from build123d import *

# Parameters (mm, degrees)
F1_DEPTH = 38.1
F3_DEPTH = 28.448
F4_R     = 7.112
F5_DEPTH = 27.178
F6_R     = 8.001
F7_DEPTH = 28.448


with BuildPart() as f1:
    # F0 (on Top) → F1 (new body)
    with BuildSketch(Plane.XY):
        Polygon((-15.113, 0), (0, 0), (15.113, 0), (15.113, -38.1), (20.574, -38.1), (20.574, -53.848), (28.448, -53.848), (28.448, 11.43), (12.7, 27.178), (0, 27.178), (-12.7, 27.178), (-28.448, 11.43), (-28.448, -53.848), (-20.574, -53.848), (-20.574, -38.1), (-15.113, -38.1), align=None)
    extrude(amount=F1_DEPTH)

    # F2 (on Right) → F3 (cut, symmetric)
    with BuildSketch(Plane.YZ):
        Polygon((27.178, 38.1), (11.43, 38.1), (27.178, 29.0068), align=None)
        Polygon((27.178, 9.0932), (11.43, 0), (27.178, 0), align=None)
    extrude(amount=F3_DEPTH, both=True, mode=Mode.SUBTRACT)

    # F4 (on face) → F5 (cut)
    with BuildSketch(Plane(origin=(0, 27.178, 0), x_dir=(-1, 0, 0), z_dir=(0, 1, 0))):
        with Locations((0, 19.05)):
            Circle(F4_R)
    extrude(amount=-F5_DEPTH, mode=Mode.SUBTRACT)

    # F6 (on Right) → F7 (cut, symmetric)
    with BuildSketch(Plane.YZ):
        with Locations((-22.352, 19.05)):
            Circle(F6_R)
        with BuildLine():
            ThreePointArc((-53.848, 23.876), (-39.346733, 33.748623), (-22.352, 38.1))
            Line((-22.352, 38.1), (-53.848, 38.1))
            Line((-53.848, 38.1), (-53.848, 23.876))
        make_face()
    extrude(amount=F7_DEPTH, both=True, mode=Mode.SUBTRACT)


solid = f1.part
Build history of the part. All positions in model axes, mm. A direction names the side the tool comes from. Coordinates: 2 decimals unless noted, no trailing zeros. Order: outer loops, then holes, each group sorted by start corner. A loop starts at its lowest first (then second) coordinate and runs counter-clockwise, first axis right, second up. Notation, with made-up numbers: (-40, -11) -> (-33, -11) arc R14 ccw to (-33, -2) -> close; hole circle Ø3 at (78.25, 88). An arc over 180 degrees is marked (long way). One line per item, written item: value.
(1) Tool access for faces 4 (the flat face through (20.574, -46, 17)), 5 (the flat face through (-25, -53.848, 12)): list every direction of +Z, -Z, +X, -X, +Y, -Y with a clear straight run to the whole face (end or side of a thin tool).
Checked values:
face 4: +Z, -Z, -Y
face 5: +Z, -Z, +X, -X, -Y
(2) Slice it at C-C, the plane y = -24. List the corners of the cut face in (x, z), plus the area to 3 significant figures.
Checked values:
outline: (-28.45, 0) -> (-15.11, 0) -> (-15.11, 11.22) -> (-28.45, 11.22) -> close; (-28.45, 26.88) -> (-15.11, 26.88) -> (-15.11, 37.95) -> (-28.45, 37.95) -> close; (15.11, 0) -> (28.45, 0) -> (28.45, 11.22) -> (15.11, 11.22) -> close; (15.11, 26.88) -> (28.45, 26.88) -> (28.45, 37.95) -> (15.11, 37.95) -> close
area: 594 mm2
(3) Probe line 1 (X direction, y = -5, z = 30); line 2 (X direction, y = -40, z = 10); line 3 (Y direction, x = -26, z = 17). List the from-to ranges inside material, lowest first. Write a range as [from, to].
Checked values:
line 1: [-28.45, -15.11], [15.11, 28.45]
line 2: [-28.45, -20.57], [20.57, 28.45]
line 3: [-53.85, -30.09], [-14.62, 13.88]
(4) Slice it at A-A, the plane z = 19.05. List the corners of the cut face in (x, y), plus the area to 3 significant figures.
Checked values:
outline: (-28.45, -53.85) -> (-20.57, -53.85) -> (-20.57, -38.1) -> (-15.11, -38.1) -> (-15.11, -30.35) -> (-28.45, -30.35) -> close; (-28.45, -14.35) -> (-15.11, -14.35) -> (-15.11, 0) -> (-7.11, 0) -> (-7.11, 27.18) -> (-12.7, 27.18) -> (-28.45, 11.43) -> close; (7.11, 0) -> (15.11, 0) -> (15.11, -14.35) -> (28.45, -14.35) -> (28.45, 11.43) -> (12.7, 27.18) -> (7.11, 27.18) -> close; (15.11, -38.1) -> (20.57, -38.1) -> (20.57, -53.85) -> (28.45, -53.85) -> (28.45, -30.35) -> (15.11, -30.35) -> close
area: 1,750 mm2
(5) Mould opens along X. For faces 1 (the flat face through (0, 1, 0)), 2 (the flat face through (-15.113, -15, 15)), 3 (the flat face through (-22.214, 17.664, 18.783)) say: pulls with the +X half, pulls with the -X half, needs draft (parallel to the pull), parting line crosses it, or undercut.
Checked values:
face 1: needs draft
face 2: undercut
face 3: pulls with the -X half
(6) Slice it at B-B, the plane x = 0. List the corners of the cut face in (y, z).
Checked values:
outline: (0, 0) -> (11.43, 0) -> (27.18, 9.09) -> (27.18, 11.94) -> (0, 11.94) -> close; (0, 26.16) -> (27.18, 26.16) -> (27.18, 29.01) -> (11.43, 38.1) -> (0, 38.1) -> close
(7) Slice it at D-D, the plane x = -24. List the corners of the cut face in (y, z), plus the area to 3 significant figures.
Checked values:
outline: (-53.85, 0) -> (11.43, 0) -> (15.88, 2.57) -> (15.88, 35.53) -> (11.43, 38.1) -> (-22.35, 38.1) arc R50.8 ccw to (-53.85, 23.88) -> close; hole circle Ø16 at (-22.35, 19.05)
area: 2,290 mm2
(8) Drop flat-ended pins along their axis: pin 1 Ø2 at (x, y) = (12.5, -32.5) entering from +Z; pin 2 Ø4 at (x, z) = (5.5, 27) entering from -Y; pin 3 Ø4.5 at (x, z) = (18, 9) entering from -Y. Give the stop position or say it passes through.
Checked values:
pin 1: through
pin 2: y = 0
pin 3: y = -38.1
